Autodesk Inventor part; units mm, degrees
ref_plane "YZ Plane" through (0, 0, 0) normal (1, 0, 0) x (0, 1, 0)
ref_plane "XZ Plane" through (0, 0, 0) normal (0, 1, 0) x (-1, 0, 0)
ref_plane "XY Plane" through (0, 0, 0) normal (0, 0, 1) x (1, 0, 0)
sketch "Sketch1" plane through (0, 0, 0) normal (0, 1, 0) x (-1, 0, 0)
  circle A0 centre (0, 0) radius 2.0955
  circle A1 centre (0, -129.1082) radius 2.0955
  arc A2 (4.7625, 0) -> (-4.7625, 0) centre (0, 0) ccw
  arc A3 (-4.7625, -129.1082) -> (4.7625, -129.1082) centre (0, -129.1082) ccw
  line L0 (4.7625, 0) -> (4.7625, -129.1082)
  line L1 (-4.7625, -129.1082) -> (-4.7625, 0)
  dimension "d0" = 4.191
  dimension "d1" = 4.191
  dimension "d2" = 9.525
  dimension "d3" = 9.525
extrude "Extrusion1" add sketch "Sketch1" along normal blind 1.5875
equation "\"BendRadius\" = Thickness"
equation "\"BendReliefWidth\" = Thickness"
equation "\"BendReliefDepth\" = 0.5 * Thickness"
equation "\"CornerReliefSize\" = 4 * Thickness"
equation "\"MinimumRemnant\" = 2 * Thickness"
equation "\"TransitionRadius\" = BendRadius"
equation "\"JacobiRadiusSize\" = BendRadius"
equation "\"GapSize\" = Thickness"
properties part number "brace-gussest" material "Acetal Resin, Black"
Check sheet for the modelled part. Datum: model origin and axes. Units: mm. Round coordinates to 2 decimals unless told otherwise and drop trailing zeros. Write each loop counter-clockwise with the first axis right and the second up, starting at its lowest first coordinate (ties: lowest second). Pieces come first, ordered by that corner, then holes. Notation, with made-up numbers: (8, 63.25) - (42, 63.25) arc R20 cw to (42, 96.25) - close; hole circle Ø4 at (66, 11.5). An arc over 180 degrees is marked (long way). Return JSON: item names as keys, results as strings.
Q1. Cross-section at B-B (y = 0.6). Record the boundary of the cut face in (x, z) (1 decimal), then the cut area to 3 significant figures.
Returned:
{"outline": "(-4.8, -129.1) arc R4.8 ccw to (4.8, -129.1) - (4.8, 0) arc R4.8 ccw to (-4.8, 0) - close; hole circle Ø4.2 at (0, -129.1); hole circle Ø4.2 at (0, 0)", "area": "1,270 mm²"}
Q2. Cross-section at A-A (x = 0). Record the boundary of the cut face in (y, z).
Returned:
{"outline": "(0, -133.87) - (1.59, -133.87) - (1.59, -131.2) - (0, -131.2) - close; (0, -127.01) - (1.59, -127.01) - (1.59, -2.1) - (0, -2.1) - close; (0, 2.1) - (1.59, 2.1) - (1.59, 4.76) - (0, 4.76) - close"}
Q3. Depth check by flat-ended pin: P1, Ø1.5, axis at x = 2, z = -55, coming from the -Y side; P2, Ø4, axis at x = 0, z = -129.11, coming from the -Y side. Enter the tip coordinate at first touch or a pass-through.
Returned:
{"P1": "stops at y = 0", "P2": "passes through"}
Q4. Draft check along Z on faces 1 (the flat face through (0, 1.588, -64)), 2 (the cylindrical face through (0.45, 0.78, -127.06)), 3 (the cylindrical face through (0.1, 0.78, 4.76)). Enter one of: released by +Z, released by -Z, zero draft, split by the parting line, or undercut.
Returned:
{"face 1": "zero draft", "face 2": "undercut", "face 3": "released by +Z"}
Q5. Scan lines: L1, parallel to Z at x = 0, y = 1.1; L2, parallel to Z at x = -1, y = 1.4; L3, parallel to X at y = 1.4, z = -1. Record each from-to range of solid material in increasing order. Write a range as from..to.
Returned:
{"L1": "z = -133.87..-131.2, -127.01..-2.1, 2.1..4.76", "L2": "z = -133.76..-130.95, -127.27..-1.84, 1.84..4.66", "L3": "x = -4.76..-1.84, 1.84..4.76"}
